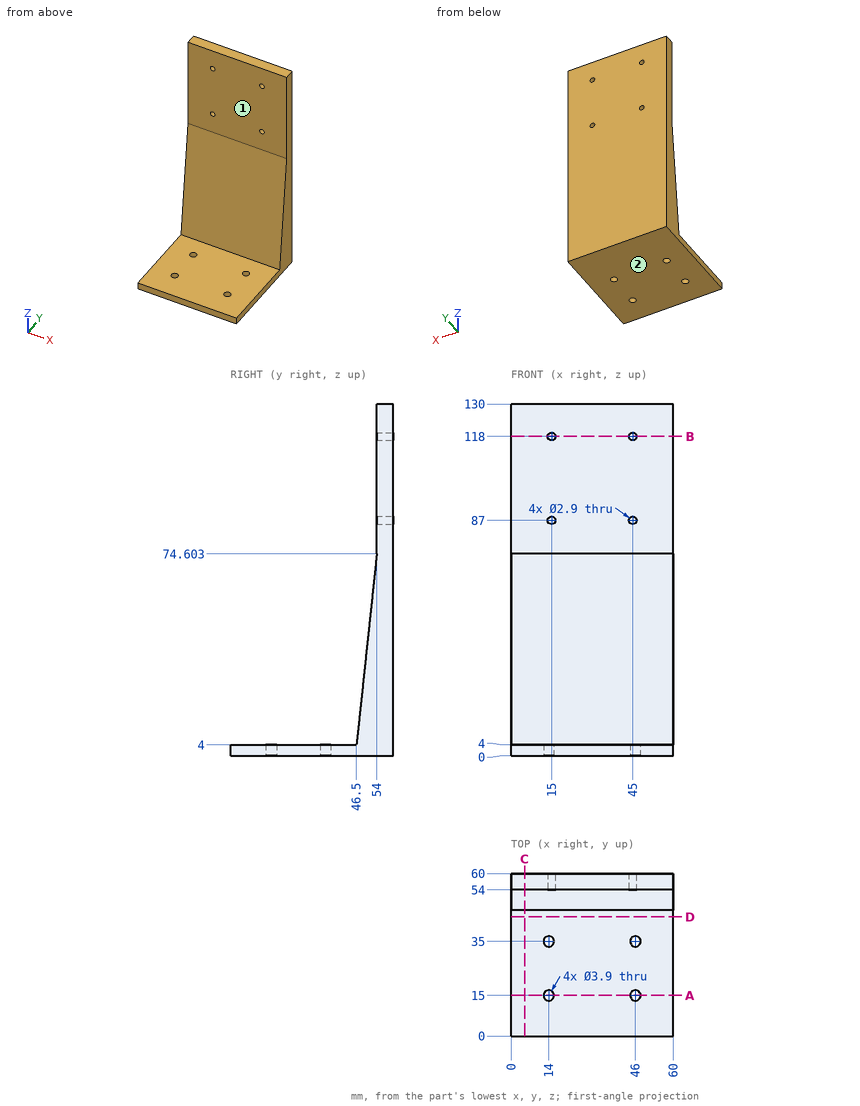
Answer from the drawing. Dimensions are ordinates in mm from the lowest x, y and z of the part. A direction names the side the tool comes from. Coordinates: 2 decimals unless noted, no trailing zeros. Loops run counter-clockwise (first coordinate to the right, second up) from the corner with the lowest first, then second, coordinate; pieces in that order, holes last.
1) Section A-A (y = 15) is taken. Give the vertices of the cut face in (x, z).
Results:
outline: (0, 0) - (12.05, 0) - (12.05, 4) - (0, 4) - close; (15.95, 0) - (44.05, 0) - (44.05, 4) - (15.95, 4) - close; (47.95, 0) - (60, 0) - (60, 4) - (47.95, 4) - close
2) Section D-D (y = 44) is taken. Give the vertices of the cut face in (x, z), plus the area to 3 significant figures.
Results:
outline: (0, 0) - (60, 0) - (60, 4) - (0, 4) - close
area: 240 mm2
3) Flat-ended cylindrical pins translate along their axes: pin 1 (6 mm diameter, centred on x = 46, y = 15, fed in from +Z); pin 2 (16.5 mm diameter, centred on x = 20.5, z = 93, fed in from -Y); pin 3 (8 mm diameter, centred on x = 16, z = 33.5, fed in from -Y). Find the tip coordinate at first contact, or state that the pin passes through.
Results:
pin 1: stops at z = 4
pin 2: stops at y = 54
pin 3: stops at y = 49.21
4) For the marked faces 1 and 2, determine the directions among +Z, -Z, +X, -X, +Y, -Y from which every point of the face is accessible in a straight line to the end or side of a thin tool.
Results:
face 1: +Z, +X, -X, -Y
face 2: -Z, +X, -X, +Y, -Y
5) Consider probe 1 along Y at (x, z) = (46, 2); probe 2 along X at (y, z) = (56.25, 118); probe 3 along Z at (x, y) = (15, 58). Determine where each line is inside the solid, lowest interval first.
Results:
probe 1: y = 0 to 13.05, 16.95 to 33.05, 36.95 to 60
probe 2: x = 0 to 13.55, 16.45 to 43.55, 46.45 to 60
probe 3: z = 0 to 85.55, 88.45 to 116.55, 119.45 to 130
6) Section B-B (z = 118) is taken. Give the vertices of the cut face in (x, y).
Results:
outline: (0, 54) - (13.55, 54) - (13.55, 60) - (0, 60) - close; (16.45, 54) - (43.55, 54) - (43.55, 60) - (16.45, 60) - close; (46.45, 54) - (60, 54) - (60, 60) - (46.45, 60) - close
7) Section C-C (x = 5) is taken. Give the vertices of the cut face in (y, z), plus the area to 3 significant figures.
Results:
outline: (0, 0) - (60, 0) - (60, 130) - (54, 130) - (54, 74.6) - (46.5, 4) - (0, 4) - close
area: 1,260 mm2
